Check sheet for the modelled part. Datum: model origin and axes. Units: mm. Face numbers are marked on the shaded views. A direction names the side the tool comes from. Give positions to 0.01 mm unless a question says otherwise; leave off trailing zeros. Order: outer loops, then holes, each group sorted by start corner. A loop starts at its lowest first (then second) coordinate and runs counter-clockwise, first axis right, second up. Notation, with made-up numbers: (84.5, 80) -> (99.5, 80) arc R20 cw to (99.5, 114) -> close; hole circle Ø2 at (32, -9.75). An arc over 180 degrees is marked (long way). One line per question, with ' | ' between items.
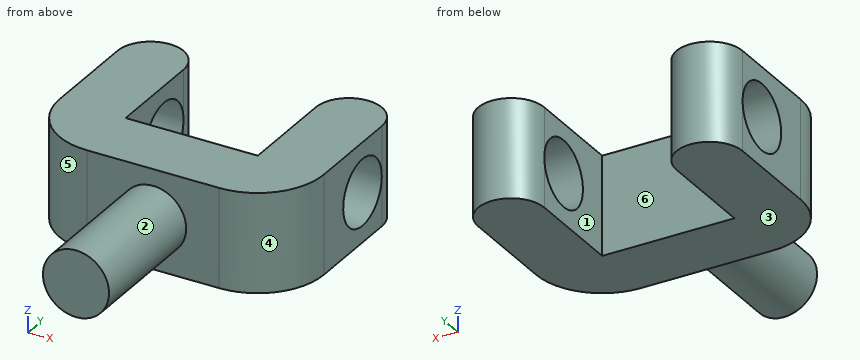
```python
from build123d import *

# Parameters (mm, degrees)
BOSS_EXTRUDE1_DEPTH = 7.5
SKETCH3_R           = 5
BOSS_EXTRUDE2_DEPTH = 20
FILLET1_R           = 10
SKETCH2_R           = 5
CUT_EXTRUDE1_DEPTH  = 40


with BuildPart() as part:
    # Sketch1 → Boss-Extrude1 (new body, symmetric)
    with BuildSketch(Plane.XY):
        with BuildLine():
            Line((10, 5), (10, 20))
            ThreePointArc((10, 20), (15, 25), (20, 20))
            Line((20, 20), (20, -5))
            Line((20, -5), (-20, -5))
            Line((-20, -5), (-20, 20))
            ThreePointArc((-20, 20), (-15, 25), (-10, 20))
            Line((-10, 20), (-10, 5))
            Line((-10, 5), (10, 5))
        make_face()
    extrude(amount=BOSS_EXTRUDE1_DEPTH, both=True)

    # Sketch3 → Boss-Extrude2 (add)
    with BuildSketch(Plane.XZ.offset(5)):
        Circle(SKETCH3_R)
    extrude(amount=BOSS_EXTRUDE2_DEPTH)

    # Fillet1
    fillet1_edges = [part.edges().sort_by_distance(p)[0] for p in [
        (20, -5, 0),
        (-20, -5, 0),
    ]]
    fillet(fillet1_edges, radius=FILLET1_R)

    # Sketch2 → Cut-Extrude1 (cut)
    with BuildSketch(Plane(origin=(20, 0, 0), x_dir=(0, 0, -1), z_dir=(1, 0, 0))):
        with Locations((0, 15)):
            Circle(SKETCH2_R)
    extrude(amount=-CUT_EXTRUDE1_DEPTH, mode=Mode.SUBTRACT)


solid = part.part
```
Q1. Section check B-B (x = 0). Enter the section's corners in (y, z).
Result sheet:
outline: (-25, -5) -> (-5, -5) -> (-5, -7.5) -> (5, -7.5) -> (5, 7.5) -> (-5, 7.5) -> (-5, 5) -> (-25, 5) -> close
Q2. Thickness scan on line 1 (Z direction, x = -13, y = 15); line 2 (X direction, y = 8.5, z = 2.25); line 3 (Y direction, x = 2.5, z = 0.5). Record the ranges inside material, lowest first.
Result sheet:
line 1: z = -7.5 to -5, 5 to 7.5 | line 2: x = -20 to -10, 10 to 20 | line 3: y = -25 to 5
Q3. Section check D-D (x = 16). Enter the section's corners in (y, z).
Result sheet:
outline: (-3, -7.5) -> (24.9, -7.5) -> (24.9, 7.5) -> (-3, 7.5) -> close; hole circle Ø10 at (15, 0)
Q4. Mould release check, pull along X, two halves, no side actions. Record for the marked faces 4, 5 and 6: pulls with the +X half, pulls with the -X half, needs draft (parallel to the pull), parting line crosses it, or undercut.
Result sheet:
face 4: pulls with the +X half | face 5: pulls with the -X half | face 6: undercut
Q5. Section check C-C (z = -6.5). Enter the section's corners in (x, y), and give its area (3 significant figures).
Result sheet:
outline: (-20, 5) arc R10 ccw to (-10, -5) -> (10, -5) arc R10 ccw to (20, 5) -> (20, 20) arc R5 ccw to (10, 20) -> (10, 5) -> (-10, 5) -> (-10, 20) arc R5 ccw to (-20, 20) -> close | area: 736 mm2
Q6. Depth check by flat-ended pin: pin 1 Ø1.5 at (y, z) = (3.5, 0.5) entering from +X; pin 2 Ø7.5 at (x, z) = (-3.5, 1) entering from +Y; pin 3 Ø6 at (x, z) = (11, 4) entering from +Y. Enter the tip coordinate at first touch or a pass-through.
Result sheet:
pin 1: stops at x = 19.97 | pin 2: stops at y = 5 | pin 3: stops at y = 24.9
Q7. Access from +Z, -Z, +X, -X, +Y, -Y to the whole of each face (thin tool, end or side, straight path). Record for the marked faces 1, 2 and 3.
Result sheet:
face 1: +Z, -Z, +Y | face 2: -Y | face 3: -Z, +X, -X, +Y, -Y
Q8. Section check A-A (z = 4). Enter the section's corners in (x, y), and give its area (3 significant figures).
Result sheet:
outline: (-20, 5) arc R10 ccw to (-10, -5) -> (-3, -5) -> (-3, -25) -> (3, -25) -> (3, -5) -> (10, -5) arc R10 ccw to (20, 5) -> (20, 12) -> (10, 12) -> (10, 5) -> (-10, 5) -> (-10, 12) -> (-20, 12) -> close; (-20, 18) -> (-10, 18) -> (-10, 20) arc R5 ccw to (-20, 20) -> close; (10, 18) -> (20, 18) -> (20, 20) arc R5 ccw to (10, 20) -> close | area: 736 mm2
